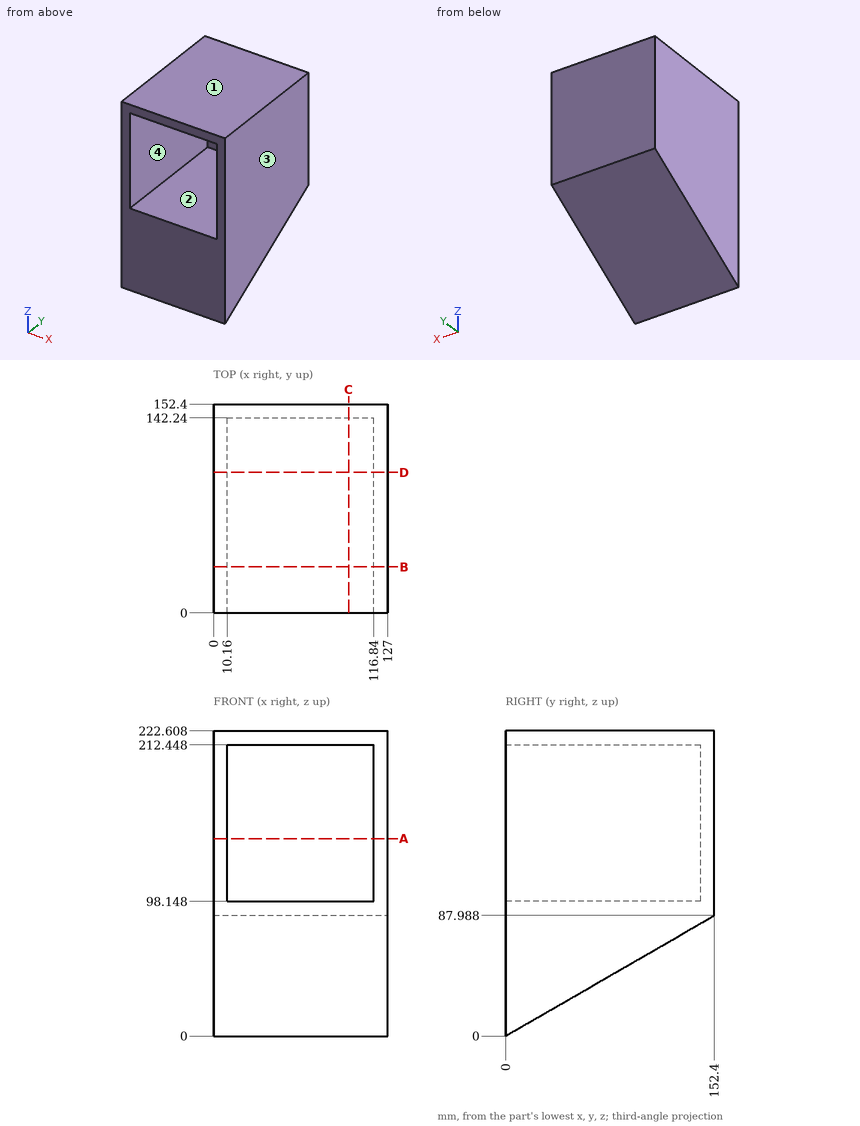
Could you check a few things on this drawing? It's one solid part, dimensions in mm from its lowest x, y, z. Coordinates: 2 decimals unless noted, no trailing zeros. Loops run counter-clockwise (first coordinate to the right, second up) from the corner with the lowest first, then second, coordinate; pieces in that order, holes last. Notation, with made-up numbers: (-2.75, -26.5) - (37.25, -26.5) arc R20 ccw to (37.25, -0.5) - close; hole circle Ø3 at (25, 37). An arc over 180 degrees is marked (long way). Answer as a JSON object with one key per item and string values. Group by question number.
Item 1: If we section it at A-A (z = 144): List the corners of the cut face in (x, y) for me.
Item 2: If I drill on L1, parallel to X at y = 43, z = 176; L2, parallel to Y at x = 33, z = 187; L3, parallel to Z at x = 37.5, y = 69.5, over which ranges is the centre line in solid material (lowest first)? Write a range as from..to.
Item 3: If we section it at B-B (y = 33.5): List the corners of the cut face in (x, z) for me, plus the area to 3 significant figures.
Item 4: If we section it at D-D (y = 102.5): List the corners of the cut face in (x, z) for me, plus the area to 3 significant figures.
Item 5: If we section it at C-C (x = 98.5): List the corners of the cut face in (y, z) for me.
Item 6: If we mould it in two halves opening along Z, with no side actions, what happens to the marked faces 1, 2, 3 and 4? For each: released by +Z, released by -Z, zero draft, split by the parting line, or undercut.
Item 7: For pin 1 (4 mm diameter, centred on x = 41.5, z = 158, fed in from -Y); pin 2 (4 mm diameter, centred on x = 43, z = 80, fed in from +Y), each with a flat end and sliding along its axis, tell me the tip position at first contact or that it passes through.
Returned:
{
 "1": {"outline": "(0, 0) - (10.16, 0) - (10.16, 142.24) - (116.84, 142.24) - (116.84, 0) - (127, 0) - (127, 152.4) - (0, 152.4) - close"},
 "2": {"L1": "x = 0..10.16, 116.84..127", "L2": "y = 142.24..152.4", "L3": "z = 40.13..98.15, 212.45..222.61"},
 "3": {"outline": "(0, 19.34) - (127, 19.34) - (127, 222.61) - (0, 222.61) - close; hole (10.16, 98.15) - (116.84, 98.15) - (116.84, 212.45) - (10.16, 212.45) - close", "area": "13,600 mm²"},
 "4": {"outline": "(0, 59.18) - (127, 59.18) - (127, 222.61) - (0, 222.61) - close; hole (10.16, 98.15) - (116.84, 98.15) - (116.84, 212.45) - (10.16, 212.45) - close", "area": "8,560 mm²"},
 "5": {"outline": "(0, 0) - (152.4, 87.99) - (152.4, 222.61) - (0, 222.61) - (0, 212.45) - (142.24, 212.45) - (142.24, 98.15) - (0, 98.15) - close"},
 "6": {"face 1": "released by +Z", "face 2": "undercut", "face 3": "zero draft", "face 4": "undercut"},
 "7": {"pin 1": "stops at y = 142.24", "pin 2": "stops at y = 142.03"}
}
